Check sheet for the modelled part. Datum: model origin and axes. Units: mm. A direction names the side the tool comes from. Round coordinates to 2 decimals unless told otherwise and drop trailing zeros. Loops run counter-clockwise (first coordinate to the right, second up) from the corner with the lowest first, then second, coordinate; pieces in that order, holes last. Notation, with made-up numbers: M 56.25,-21.75 L 76.25,-21.75 A29 ccw 76.25,10.25 Z; hole C -36.75,8 d2. An arc over 180 degrees is marked long. Write item = value, one per line. Start each with the question number.
(1) Scan lines: L1, parallel to X at y = -3, z = 9.5; L2, parallel to Z at x = 7, y = -35; L3, parallel to Z at x = 25.5, y = -63. Record each from-to range of solid material in increasing order. Write a range as from..to.
(2) Cross-section at D-D on x = 11.5. Record the boundary of the cut face in (y, z).
(3) Cross-section at C-C on z = 16. Record the boundary of the cut face in (x, y).
(4) Set-up check for faces 1 (the face through (11, -38, 14.557)), 2 (the face through (21, -77.216, 11)): record each of +Z, -Z, +X, -X, +Y, -Y from which the full face is reachable in a straight line by a thin tool's end or side.
(5) Go/stop test with flat-tipped pins: P1, Ø1.5, axis at y = -35.5, z = 17, coming from the -X side; P2, Ø10.5, axis at x = 15, y = -31.5, coming from the +Z side; P3, Ø1.5, axis at x = 25, y = -26, coming from the +Z side. Record where each tip stops, or that it passes through.
(6) Cross-section at B-B on y = -8. Record the boundary of the cut face in (x, z).
(7) Cross-section at A-A on x = 26.5. Record the boundary of the cut face in (y, z).
from build123d import *

# Parameters (mm, degrees)
F1_DEPTH = 77.216
F2_R     = 12.7
F3_R     = 4.324239
F4_DEPTH = 77.216


with BuildPart() as f1:
    # F0 (on Front) → F1 (new body)
    with BuildSketch(Plane.XZ):
        Polygon((0, 14.556793), (0, 0), (34.454569, 0), (34.454569, 39.271925), (21.049753, 27.33326), (21.049753, 14.556793), align=None)
    extrude(amount=F1_DEPTH)

    # F2
    f2_edges = [f1.edges().sort_by_distance(p)[0] for p in [
        (21.049753, -38.608, 27.33326),
    ]]
    fillet(f2_edges, radius=F2_R)

    # F3 (on face) → F4 (cut, through all)
    with BuildSketch(Plane.XZ.offset(77.216)):
        with Locations((24.158696, 6.31389)):
            Circle(F3_R)
    extrude(amount=-F4_DEPTH, mode=Mode.SUBTRACT)


solid = f1.part
Result:
q1.L1 = 0..21.24, 27.08..34.45
q1.L2 = 0..14.56
q1.L3 = 0..2.2, 10.42..31.3
q2.outline = M -77.22,0 L 0,0 L 0,14.56 L -77.22,14.56 Z
q3.outline = M 21.05,-77.22 L 34.45,-77.22 L 34.45,0 L 21.05,0 Z
q4.face_1 = +Z, -X, +Y, -Y
q4.face_2 = +Z, -Z, +X, -X, -Y
q5.P1 = 21.05
q5.P2 = 14.56
q5.P3 = 31.52
q6.outline = M 0,0 L 34.45,0 L 34.45,39.27 L 25.3,31.12 A12.7 ccw 21.05,21.64 L 21.05,14.56 L 0,14.56 Z; hole C 24.16,6.31 d8.65
q7.outline = M -77.22,0 L 0,0 L 0,2.68 L -77.22,2.68 Z; M -77.22,9.95 L 0,9.95 L 0,32.19 L -77.22,32.19 Z
